Geometry check sheet. Reference: the model listing, model coordinates, mm. A direction names the side the tool comes from. Coordinates: 2 decimals unless noted, no trailing zeros. Order: outer loops, then holes, each group sorted by start corner. A loop starts at its lowest first (then second) coordinate and runs counter-clockwise, first axis right, second up. Notation, with made-up numbers: (79.5, 23) - (107.5, 23) arc R12 cw to (107.5, 41) - close; hole circle Ø4 at (71, -37). An arc over 180 degrees is marked (long way). One line per item, written item: value. Start each with the question number.
```python
from build123d import *

# Parameters (mm, degrees)
SKETCH_1_R          = 2.55
SKETCH_1_R_2        = 3.6
SKETCH_1_R_3        = 2.25
SKETCH_1_R_4        = 1.75
EXTRUDE_1_DEPTH     = 4
SKETCH_2_W          = 60.730368491
SKETCH_2_H          = 80
CUT_EXTRUDE_1_DEPTH = 10
FILLET_1_R          = 20


with BuildPart() as part:
    # 草图1 → 凸台-拉伸1 (new body)
    with BuildSketch(Plane.XY):
        with BuildLine():
            ThreePointArc((-133.333333333, 151.160446029), (-150.358269338, 147.855332986), (-148.948414541, 130.569948187))
            ThreePointArc((-148.948414541, 130.569948187), (-92.849538953, 0), (-148.948414541, -130.569948187))
            ThreePointArc((-148.948414541, -130.569948187), (-150.358269338, -147.855332986), (-133.333333333, -151.160446029))
            ThreePointArc((-133.333333333, -151.160446029), (0, -114.369366599), (133.333333333, -151.160446029))
            ThreePointArc((133.333333333, -151.160446029), (150.358269338, -147.855332986), (148.948414541, -130.569948187))
            ThreePointArc((148.948414541, -130.569948187), (92.849538953, 0), (148.948414541, 130.569948187))
            ThreePointArc((148.948414541, 130.569948187), (150.358269338, 147.855332986), (133.333333333, 151.160446029))
            ThreePointArc((133.333333333, 151.160446029), (0, 114.369366599), (-133.333333333, 151.160446029))
        make_face()
        with Locations((0, 90)):
            Circle(SKETCH_1_R, mode=Mode.SUBTRACT)
        with Locations((0, -90)):
            Circle(SKETCH_1_R_2, mode=Mode.SUBTRACT)
        with Locations((60, 90)):
            Circle(SKETCH_1_R, mode=Mode.SUBTRACT)
        with Locations((60, -90)):
            Circle(SKETCH_1_R_2, mode=Mode.SUBTRACT)
        with Locations((-60, 90)):
            Circle(SKETCH_1_R, mode=Mode.SUBTRACT)
        with Locations((-60, -90)):
            Circle(SKETCH_1_R_2, mode=Mode.SUBTRACT)
        with Locations((-140, 140)):
            Circle(SKETCH_1_R_3, mode=Mode.SUBTRACT)
        with Locations((140, 140)):
            Circle(SKETCH_1_R_3, mode=Mode.SUBTRACT)
        with Locations((-140, -140)):
            Circle(SKETCH_1_R_3, mode=Mode.SUBTRACT)
        with Locations((140, -140)):
            Circle(SKETCH_1_R_3, mode=Mode.SUBTRACT)
        with Locations((-35, 8)):
            Circle(SKETCH_1_R_4, mode=Mode.SUBTRACT)
        with Locations((35, 8)):
            Circle(SKETCH_1_R_4, mode=Mode.SUBTRACT)
        with Locations((0, 110)):
            Circle(SKETCH_1_R_4, mode=Mode.SUBTRACT)
    extrude(amount=EXTRUDE_1_DEPTH)

    # 草图2 → 切除-拉伸1 (cut)
    with BuildSketch(Plane.XY.offset(4)):
        with Locations((-90.365184246, 0)):
            Rectangle(SKETCH_2_W, SKETCH_2_H)
        with Locations((90.365184246, 0)):
            Rectangle(SKETCH_2_W, SKETCH_2_H)
    extrude(amount=-CUT_EXTRUDE_1_DEPTH, mode=Mode.SUBTRACT)

    # 圆角1
    fillet_1_edges = [part.edges().sort_by_distance(p)[0] for p in [
        (60, -40, 2),
        (60, 40, 2),
        (-97.350251205, -40, 2),
        (-97.350251205, 40, 2),
        (-60, 40, 2),
        (-60, -40, 2),
        (97.350251205, 40, 2),
        (97.350251205, -40, 2),
    ]]
    fillet(fillet_1_edges, radius=FILLET_1_R)


solid = part.part
```
Q1. Gauge pin test, flat ends, axial feed: P1, Ø1, axis at x = 81, z = 1, coming from the -Y side; P2, Ø6, axis at x = -9.5, y = 115, coming from the +Z side; P3, Ø1.6, axis at x = -81.5, z = 2.5, coming from the -Y side; P4, Ø1, axis at x = 83.5, z = 0.5, coming from the -Y side. Record the tip position at first contact, or that the pin passes through.
Q2. Set-up check for faces 4 (the cylindrical face through (-150.52, -147.64, 1.97)), 5 (the cylindrical face through (-119.83, -94.79, 1.97)), 6 (the cylindrical face through (65.703, -33.986, 1.972)): record each of +Z, -Z, +X, -X, +Y, -Y from which the full face is reachable in a straight line by a thin tool's end or side.
Q3. Cross-section at D-D, the plane x = -108.5. Enter the section's corners in (y, z), and give its area (3 significant figures).
Q4. Release check for a two-part mould opening along Y. For faces 1 (the flat face through (-2, 2, 4)), 2 (the cylindrical face through (-66.014, 34.297, 1.972)), 3 (the cylindrical face through (-1.96, -114.377, 1.972)) record: released by +Y, released by -Y, zero draft, split by the parting line, or undercut.
Q5. Cross-section at A-A, the plane x = 116. Enter the section's corners in (y, z).
Q6. Cross-section at B-B, the plane z = 3.05. Count the separate pieces of the cut face and the enclosed holes in it, and give its area (3 significant figures).
Q7. Material ranges on probe 1 along X at (y, z) = (140, 2.6); probe 2 along Y at (x, z) = (-122, 1.3); probe 3 along Y at (x, z) = (35, 2.65), recorded low to high.
Q8. Cross-section at C-C, the plane y = -1.5. Enter the section's corners in (x, z), and give its area (3 significant figures).
Check result:
1. P1: stops at y = -127.47
1. P2: stops at z = 4
1. P3: stops at y = -127.74
1. P4: stops at y = -128.31
2. face 4: +Z, -Z
2. face 5: +Z, -Z, -X
2. face 6: +Z, -Z, +X
3. outline: (-138.09, 0) - (-73.41, 0) - (-73.41, 4) - (-138.09, 4) - close; (73.41, 0) - (138.09, 0) - (138.09, 4) - (73.41, 4) - close
3. area: 517 mm2
4. face 1: zero draft
4. face 2: undercut
4. face 3: released by -Y
5. outline: (-141.68, 0) - (-88.31, 0) - (-88.31, 4) - (-141.68, 4) - close; (88.31, 0) - (141.68, 0) - (141.68, 4) - (88.31, 4) - close
6. separate pieces: 1
6. enclosed holes: 13
6. area: 51,200 mm2
7. probe 1: x = -153 to -142.25, -137.75 to -112.57, 112.57 to 137.75, 142.25 to 153
7. probe 2: y = -144.77 to -98.21, 98.21 to 144.77
7. probe 3: y = -116.74 to 6.25, 9.75 to 116.74
8. outline: (-60, 0) - (60, 0) - (60, 4) - (-60, 4) - close
8. area: 480 mm2
